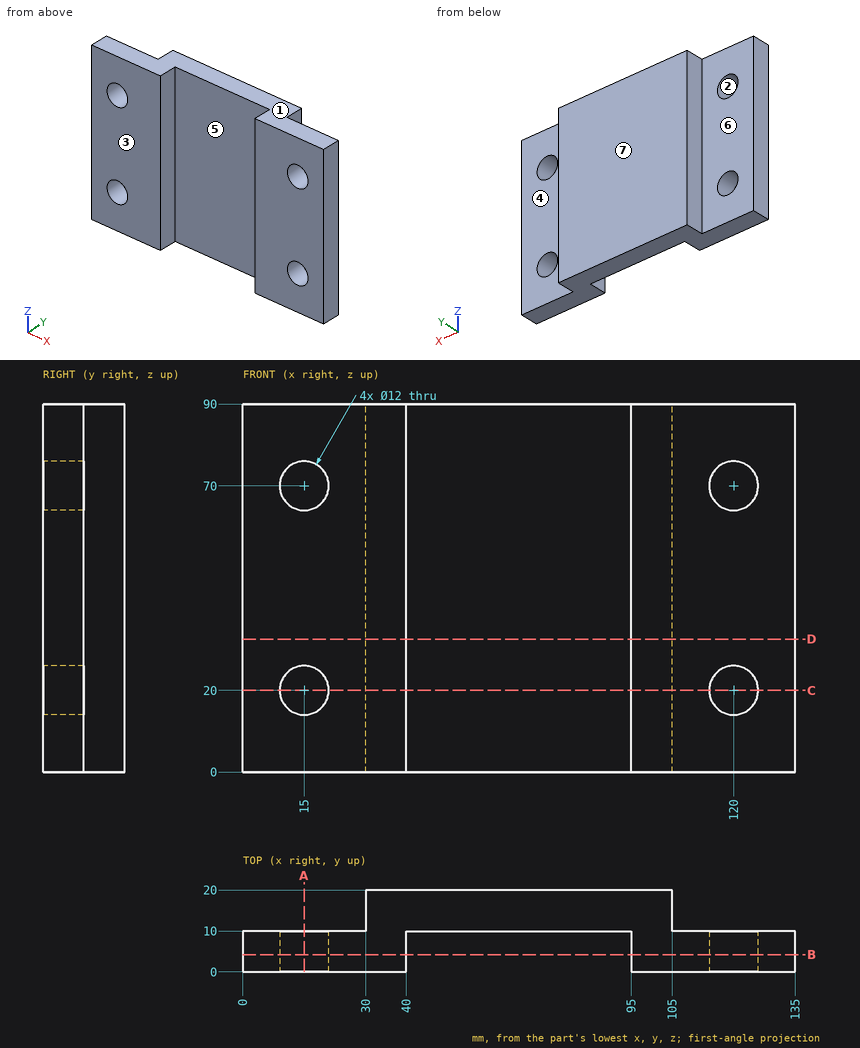
Geometry: see drawing. Coordinates: mm, zero at the bounding-box minimum. A direction names the side the tool comes from. Give positions to 0.01 mm unless a question says otherwise; leave off trailing zeros. Order: outer loops, then holes, each group sorted by start corner. A loop starts at its lowest first (then second) coordinate and runs counter-clockwise, first axis right, second up. Notation, with made-up numbers: (25.5, -17.75) - (84.5, -17.75) arc R6 ccw to (84.5, -9.75) - close; hole circle Ø6 at (38.5, 85.5). An arc over 180 degrees is marked (long way). Write each question's results on one line, items separated by ' | '.
Item 1: Draft query along Z for the marked faces 1, 2 and 3. Return one class per face: released by +Z, released by -Z, zero draft, split by the parting line, or undercut.
A:
face 1: released by +Z | face 2: undercut | face 3: zero draft
Item 2: Section C-C (z = 20). Return loops of the section in (x, y).
A:
outline: (0, 0) - (9, 0) - (9, 10) - (0, 10) - close; (21, 0) - (40, 0) - (40, 10) - (95, 10) - (95, 0) - (114, 0) - (114, 10) - (105, 10) - (105, 20) - (30, 20) - (30, 10) - (21, 10) - close; (126, 0) - (135, 0) - (135, 10) - (126, 10) - close
Item 3: Section D-D (z = 32.5). Return loops of the section in (x, y), and give its area (3 significant figures).
A:
outline: (0, 0) - (40, 0) - (40, 10) - (95, 10) - (95, 0) - (135, 0) - (135, 10) - (105, 10) - (105, 20) - (30, 20) - (30, 10) - (0, 10) - close | area: 1,550 mm^2
Item 4: Material intervals for line 1 along Z through (x, y) = (15, 4.5); line 2 along X through (y, z) = (1.5, 57); line 3 along X through (y, z) = (6.5, 73.5), sorted ascending.
A:
line 1: z = 0 to 14, 26 to 64, 76 to 90 | line 2: x = 0 to 40, 95 to 135 | line 3: x = 0 to 10.13, 19.87 to 40, 95 to 115.13, 124.87 to 135
Item 5: Section A-A (x = 15). Return loops of the section in (y, z).
A:
outline: (0, 0) - (10, 0) - (10, 14) - (0, 14) - close; (0, 26) - (10, 26) - (10, 64) - (0, 64) - close; (0, 76) - (10, 76) - (10, 90) - (0, 90) - close
Item 6: Section B-B (y = 4.25). Return loops of the section in (x, z), and give its area (3 significant figures).
A:
outline: (0, 0) - (40, 0) - (40, 90) - (0, 90) - close; (95, 0) - (135, 0) - (135, 90) - (95, 90) - close; hole circle Ø12 at (15, 20); hole circle Ø12 at (15, 70); hole circle Ø12 at (120, 20); hole circle Ø12 at (120, 70) | area: 6,750 mm^2
Item 7: Access query for the marked faces 4, 5, 6 and 7. Directions: +Z, -Z, +X, -X, +Y, -Y. A direction counts if a zero-diameter tool reaches every point of the face in a straight line with its end or side. Return the directions, or none.
A:
face 4: +Z, -Z, +X, +Y | face 5: +Z, -Z, -Y | face 6: +Z, -Z, -X, +Y | face 7: +Z, -Z, +X, -X, +Y
Item 8: Contact query for flat-ended pins moving along their axis: pin 1 Ø5 at (x, z) = (55, 48) entering from -Y; pin 2 Ø3 at (y, z) = (14.5, 23) entering from +X; pin 3 Ø24 at (x, z) = (16.5, 67.5) entering from +Y; pin 4 Ø14 at (x, z) = (15, 70) entering from -Y. Output: stop coordinate, or through.
A:
pin 1: stops at y = 10 | pin 2: stops at x = 105 | pin 3: stops at y = 10 | pin 4: stops at y = 0
